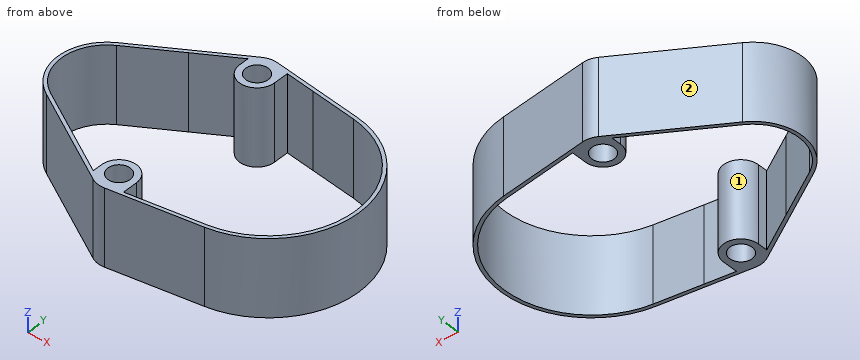
from build123d import *

# Parameters (mm, degrees)
SKETCH1_R           = 3
SKETCH1_R_2         = 4.5
SKETCH1_R_3         = 1.6
BOSS_EXTRUDE3_DEPTH = 1.6
SKETCH2_R           = 1.6
SKETCH2_R_2         = 3
SKETCH2_R_3         = 4.5
BOSS_EXTRUDE4_DEPTH = 1.5
SKETCH3_R           = 63.206562555
CUT_EXTRUDE1_DEPTH  = 1.6
SKETCH4_R           = 3
SKETCH4_R_2         = 1.6
BOSS_EXTRUDE5_DEPTH = 1.5
SKETCH5_R           = 1.6
BOSS_EXTRUDE6_DEPTH = 11
SKETCH6_R           = 49.514430464
CUT_EXTRUDE2_DEPTH  = 1.5


with BuildPart() as part:
    # Sketch1 → Boss-Extrude3 (new body)
    with BuildSketch(Plane.XY):
        with BuildLine():
            Line((12.073070054, 14.639688463), (24.958502044, 12.880515151))
            ThreePointArc((24.958502044, 12.880515151), (36.2, 0), (24.958502044, -12.880515151))
            Line((24.958502044, -12.880515151), (12.073070054, -14.639688463))
            ThreePointArc((12.073070054, -14.639688463), (11.870633815, -14.660360595), (11.66726189, -14.66726189))
            Line((11.66726189, -14.66726189), (0, -14.66726189))
            ThreePointArc((0, -14.66726189), (-0.888679088, -14.53261518), (-1.697586366, -14.140761542))
            Line((-1.697586366, -14.140761542), (-18.697586366, -2.473499652))
            ThreePointArc((-18.697586366, -2.473499652), (-19.891071988, -0.801063519), (-19.728500117, 1.247111507))
            Line((-19.728500117, 1.247111507), (-14.395762007, 12.914373397))
            ThreePointArc((-14.395762007, 12.914373397), (-13.288783625, 14.191279968), (-11.66726189, 14.66726189))
            Line((-11.66726189, 14.66726189), (11.66726189, 14.66726189))
            ThreePointArc((11.66726189, 14.66726189), (11.870633815, 14.660360595), (12.073070054, 14.639688463))
        make_face()
        Circle(SKETCH1_R, mode=Mode.SUBTRACT)
        with Locations((23.2, 0)):
            Circle(SKETCH1_R_2, mode=Mode.SUBTRACT)
        with Locations((8.6, 0)):
            Circle(SKETCH1_R, mode=Mode.SUBTRACT)
        with Locations((-17, 0)):
            Circle(SKETCH1_R_3, mode=Mode.SUBTRACT)
        with Locations((0, -11.66726189)):
            Circle(SKETCH1_R_3, mode=Mode.SUBTRACT)
        with Locations((11.66726189, -11.66726189)):
            Circle(SKETCH1_R_3, mode=Mode.SUBTRACT)
        with Locations((-11.66726189, 11.66726189)):
            Circle(SKETCH1_R_3, mode=Mode.SUBTRACT)
        with Locations((0, 11.66726189)):
            Circle(SKETCH1_R_3, mode=Mode.SUBTRACT)
        with Locations((11.66726189, 11.66726189)):
            Circle(SKETCH1_R_3, mode=Mode.SUBTRACT)
    extrude(amount=BOSS_EXTRUDE3_DEPTH)

    # Sketch2 → Boss-Extrude4 (add)
    with BuildSketch(Plane.XY.offset(1.6)):
        with BuildLine():
            Line((12.073070054, 14.639688463), (24.958502044, 12.880515151))
            ThreePointArc((24.958502044, 12.880515151), (36.2, 0), (24.958502044, -12.880515151))
            Line((24.958502044, -12.880515151), (12.073070054, -14.639688463))
            ThreePointArc((12.073070054, -14.639688463), (10.884137398, -14.56324463), (9.81871257, -14.030070687))
            Line((9.81871257, -14.030070687), (-3.080915533, -3.938014662))
            ThreePointArc((-3.080915533, -3.938014662), (-5, 0), (-3.080915533, 3.938014662))
            Line((-3.080915533, 3.938014662), (9.81871257, 14.030070687))
            ThreePointArc((9.81871257, 14.030070687), (10.884137398, 14.56324463), (12.073070054, 14.639688463))
        make_face()
        with Locations((11.66726189, 11.66726189)):
            Circle(SKETCH2_R, mode=Mode.SUBTRACT)
        Circle(SKETCH2_R_2, mode=Mode.SUBTRACT)
        with Locations((8.6, 0)):
            Circle(SKETCH2_R_2, mode=Mode.SUBTRACT)
        with Locations((23.2, 0)):
            Circle(SKETCH2_R_3, mode=Mode.SUBTRACT)
        with Locations((11.66726189, -11.66726189)):
            Circle(SKETCH2_R, mode=Mode.SUBTRACT)
    extrude(amount=BOSS_EXTRUDE4_DEPTH)

    # Sketch3 → Cut-Extrude1 (cut)
    with BuildSketch(Plane(origin=(0, 0, 0), x_dir=(-1, 0, 0), z_dir=(0, 0, -1))):
        Circle(SKETCH3_R)
    extrude(amount=-CUT_EXTRUDE1_DEPTH, mode=Mode.SUBTRACT)

    # Sketch4 → Boss-Extrude5 (add)
    with BuildSketch(Plane.XY.offset(3.1)):
        with BuildLine():
            Line((-3.602159399, 6.00203696), (10.12347929, 14.239563444))
            ThreePointArc((10.12347929, 14.239563444), (13.145208472, 14.277946455), (14.66726189, 11.66726189))
            Line((14.66726189, 11.66726189), (14.66726189, -11.66726189))
            ThreePointArc((14.66726189, -11.66726189), (13.145208472, -14.277946455), (10.12347929, -14.239563444))
            Line((10.12347929, -14.239563444), (-3.602159399, -6.00203696))
            ThreePointArc((-3.602159399, -6.00203696), (-7, 0), (-3.602159399, 6.00203696))
        make_face()
        Circle(SKETCH4_R, mode=Mode.SUBTRACT)
        with Locations((8.6, 0)):
            Circle(SKETCH4_R, mode=Mode.SUBTRACT)
        with Locations((11.66726189, 11.66726189)):
            Circle(SKETCH4_R_2, mode=Mode.SUBTRACT)
        with Locations((11.66726189, -11.66726189)):
            Circle(SKETCH4_R_2, mode=Mode.SUBTRACT)
    extrude(amount=-BOSS_EXTRUDE5_DEPTH)

    # Sketch5 → Boss-Extrude6 (add)
    with BuildSketch(Plane.XY.offset(3.1)):
        with BuildLine():
            Line((10.12347929, 14.239563444), (-3.602159399, 6.00203696))
            ThreePointArc((-3.602159399, 6.00203696), (-7, 0), (-3.602159399, -6.00203696))
            Line((-3.602159399, -6.00203696), (10.12347929, -14.239563444))
            ThreePointArc((10.12347929, -14.239563444), (11.064127193, -14.606007972), (12.073070054, -14.639688463))
            Line((12.073070054, -14.639688463), (24.958502044, -12.880515151))
            ThreePointArc((24.958502044, -12.880515151), (36.2, 0), (24.958502044, 12.880515151))
            Line((24.958502044, 12.880515151), (12.073070054, 14.639688463))
            ThreePointArc((12.073070054, 14.639688463), (11.064127193, 14.606007972), (10.12347929, 14.239563444))
        make_face()
        with Locations((11.66726189, -11.66726189)):
            Circle(SKETCH5_R, mode=Mode.SUBTRACT)
        with BuildLine():
            Line((-3.345341009, 5.573371264), (3.517564288, 9.692737701))
            Line((3.517564288, 9.692737701), (9.16726189, 13.083892566))
            Line((9.16726189, 13.083892566), (9.16726189, 11.66726189))
            ThreePointArc((9.16726189, 11.66726189), (11.66726189, 9.16726189), (14.16726189, 11.66726189))
            Line((14.16726189, 11.66726189), (14.16726189, 13.849142394))
            Line((14.16726189, 13.849142394), (18.333589211, 13.280337883))
            Line((18.333589211, 13.280337883), (24.89086735, 12.385110722))
            ThreePointArc((24.89086735, 12.385110722), (35.7, 0), (24.89086735, -12.385110722))
            Line((24.89086735, -12.385110722), (18.333589211, -13.280337883))
            Line((18.333589211, -13.280337883), (14.16726189, -13.849142394))
            Line((14.16726189, -13.849142394), (14.16726189, -11.66726189))
            ThreePointArc((14.16726189, -11.66726189), (11.66726189, -9.16726189), (9.16726189, -11.66726189))
            Line((9.16726189, -11.66726189), (9.16726189, -13.083892566))
            Line((9.16726189, -13.083892566), (3.517564288, -9.692737701))
            Line((3.517564288, -9.692737701), (-3.345341009, -5.573371264))
            ThreePointArc((-3.345341009, -5.573371264), (-6.500290279, 0), (-3.345341009, 5.573371264))
        make_face(mode=Mode.SUBTRACT)
        with Locations((11.66726189, 11.66726189)):
            Circle(SKETCH5_R, mode=Mode.SUBTRACT)
    extrude(amount=BOSS_EXTRUDE6_DEPTH)

    # Sketch6 → Cut-Extrude2 (cut)
    with BuildSketch(Plane(origin=(0, 0, 1.6), x_dir=(-1, 0, 0), z_dir=(0, 0, -1))):
        Circle(SKETCH6_R)
    extrude(amount=-CUT_EXTRUDE2_DEPTH, mode=Mode.SUBTRACT)


solid = part.part
Here's how the part is built. I have some questions about the finished solid (model axes, mm). Face numbers are marked on the shaded views. A direction names the side the tool comes from. Round coordinates to 2 decimals unless told otherwise and drop trailing zeros. Loops run counter-clockwise (first coordinate to the right, second up) from the corner with the lowest first, then second, coordinate; pieces in that order, holes last. Notation, with made-up numbers: M 56,-25 L 108,-25 A30 cw 108,9 Z; hole C 9.25,-32.75 d11. An arc over 180 degrees is marked long. Write each question's results on one line, items separated by ' | '. Start each with the question number.
(1) If I drill on probe 1 along Y at (x, z) = (12, 7.75); probe 2 along X at (y, z) = (9.5, 10.5); probe 3 along Y at (x, z) = (31.5, 3.5), over which ranges is the centre line in solid material (lowest first)? Write a range as from..to.
(2) Will these pins go through, and if not, where does the flat tip stop? P1, Ø2.5, axis at x = 11.67, y = 11.67, coming from the +Z side; P2, Ø1.5, axis at y = 6.5, z = 12, coming from the +X side; P3, Ø2, axis at y = -8.5, z = 4.5, coming from the +X side; P4, Ø1.6, axis at y = -12.5, z = 10, coming from the -X side.
(3) On a 3-axis mill with a long thin cutter (end or side, diameter ignored), from which of +Z, -Z, +X, -X, +Y, -Y can I reach the whole of each face in a straight line? I mean the marked faces 1 and 2. Say none if no direction works.
(4) I want a section at B-B (x = 19). Please give me the cut outline in (y, z).
(5) I want a section at C-C (z = 9.25). Please give me the cut outline in (x, y), then the cut area to 3 significant figures.
(6) I want a section at A-A (y = 7). Please give me the cut outline in (x, z), then the cut area to 3 significant figures.
(7) I want a section at D-D (y = 10.5). Please give me the cut outline in (x, z), then the cut area to 3 significant figures.
Solved:
1) probe 1: y = -14.65..-13.23, -10.1..-9.19, 9.19..10.1, 13.23..14.65 | probe 2: x = 2.23..3.2, 10.42..12.91, 31.32..32.07 | probe 3: y = -10.01..-9.35, 9.35..10.01
2) P1: passes through | P2: stops at x = 34.86 | P3: stops at x = 33.82 | P4: stops at x = 5.89
3) face 1: +Z, -Z | face 2: +Z, -Z, -X, +Y
4) outline: M -13.69,3.1 L -13.19,3.1 L -13.19,14.1 L -13.69,14.1 Z; M 13.19,3.1 L 13.69,3.1 L 13.69,14.1 L 13.19,14.1 Z
5) outline: M -3.6,-6 L 10.12,-14.24 A3 ccw 12.07,-14.64 L 24.96,-12.88 A13 ccw 24.96,12.88 L 12.07,14.64 A3 ccw 10.12,14.24 L -3.6,6 A7 ccw Z; hole M -3.35,-5.57 L 9.17,-13.08 L 9.17,-11.67 A2.5 cw 14.17,-11.67 L 14.17,-13.85 L 24.89,-12.39 A12.5 ccw 24.89,12.39 L 14.17,13.85 L 14.17,11.67 A2.5 cw 9.17,11.67 L 9.17,13.08 L -3.35,5.57 A6.5 ccw Z; hole C 11.67,-11.67 d3.2; hole C 11.67,11.67 d3.2 | area: 81.9 mm²
6) outline: M -1.94,3.1 L -0.97,3.1 L -0.97,14.1 L -1.94,14.1 Z; M 33.56,3.1 L 34.15,3.1 L 34.15,14.1 L 33.56,14.1 Z | area: 17.3 mm²
7) outline: M 3.89,3.1 L 4.86,3.1 L 4.86,14.1 L 3.89,14.1 Z; M 9.46,3.1 L 10.57,3.1 L 10.57,14.1 L 9.46,14.1 Z; M 12.76,3.1 L 13.88,3.1 L 13.88,14.1 L 12.76,14.1 Z; M 29.98,3.1 L 30.86,3.1 L 30.86,14.1 L 29.98,14.1 Z | area: 44.9 mm²
